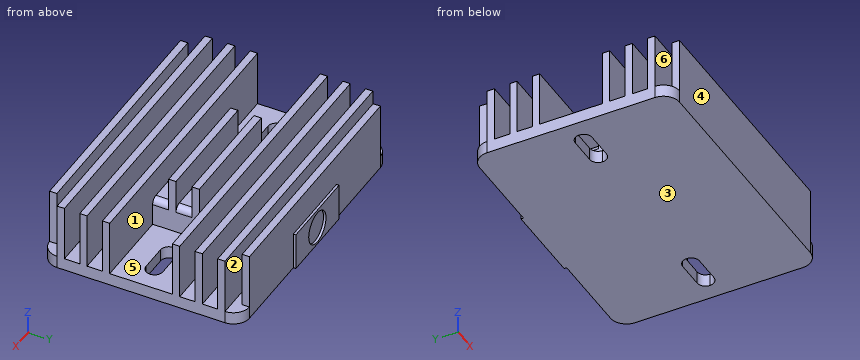
from build123d import *

# Parameters (mm, degrees)
SKETCH_1_W          = 110.2
SKETCH_1_H          = 79.6
EXTRUDE_1_DEPTH     = 4.99
SKETCH_2_W          = 52.2
SKETCH_2_H          = 6.4
EXTRUDE_2_DEPTH     = 15
SKETCH_3_W          = 46.2
SKETCH_3_H          = 73.2
EXTRUDE_3_DEPTH     = 11.2
SKETCH_4_W          = 97.6
SKETCH_4_H          = 2.9
SKETCH_4_W_2        = 46.2
SKETCH_4_W_3        = 110.2
EXTRUDE_4_DEPTH     = 22.4
SKETCH_5_W          = 17.339600334
SKETCH_5_H          = 6.7
CUT_EXTRUDE_1_DEPTH = 138.775034023
FILLET_1_R          = 3.3
FILLET_2_R          = 6.4
FILLET_3_R          = 2.5
SKETCH_6_W          = 32.2
SKETCH_6_H          = 15
EXTRUDE_5_DEPTH     = 1
SKETCH_7_R          = 6.438822501
CUT_EXTRUDE_2_DEPTH = 1


with BuildPart() as part:
    # ｽｹｯﾁ1 → ﾎﾞｽ - 押し出し1 (new body)
    with BuildSketch(Plane.XY):
        with Locations((55.1, 39.8)):
            Rectangle(SKETCH_1_W, SKETCH_1_H)
    extrude(amount=EXTRUDE_1_DEPTH)

    # ｽｹｯﾁ2 → ﾎﾞｽ - 押し出し2 (add)
    with BuildSketch(Plane.XY.offset(4.99)):
        with Locations((55.1, 76.4)):
            Rectangle(SKETCH_2_W, SKETCH_2_H)
    extrude(amount=EXTRUDE_2_DEPTH)

    # ｽｹｯﾁ3 → ﾎﾞｽ - 押し出し3 (add)
    with BuildSketch(Plane.XY.offset(4.99)):
        with Locations((55.1, 36.6)):
            Rectangle(SKETCH_3_W, SKETCH_3_H)
    extrude(amount=EXTRUDE_3_DEPTH)

    # ｽｹｯﾁ4 → ﾎﾞｽ - 押し出し4 (add)
    with BuildSketch(Plane.XY.offset(4.99)):
        with Locations((55.1, 78.15)):
            Rectangle(SKETCH_4_W, SKETCH_4_H)
        with Locations((55.1, 1.45)):
            Rectangle(SKETCH_4_W, SKETCH_4_H)
        with Locations((55.1, 44.45)):
            Rectangle(SKETCH_4_W_2, SKETCH_4_H)
        with Locations((55.1, 35.15)):
            Rectangle(SKETCH_4_W_2, SKETCH_4_H)
        with Locations((55.1, 53.75)):
            Rectangle(SKETCH_4_W_3, SKETCH_4_H)
        with Locations((55.1, 25.85)):
            Rectangle(SKETCH_4_W_3, SKETCH_4_H)
        with Locations((55.1, 71.781871857)):
            Rectangle(SKETCH_4_W_3, SKETCH_4_H)
        with Locations((55.1, 7.818128143)):
            Rectangle(SKETCH_4_W_3, SKETCH_4_H)
        with Locations((55.1, 16.834064072)):
            Rectangle(SKETCH_4_W_3, SKETCH_4_H)
        with Locations((55.1, 62.765935928)):
            Rectangle(SKETCH_4_W_3, SKETCH_4_H)
    extrude(amount=EXTRUDE_4_DEPTH)

    # ｽｹｯﾁ5 → ｶｯﾄ - 押し出し1 (cut, through all)
    with BuildSketch(Plane.XY.offset(4.99)):
        with Locations((15.05636048, 39.95)):
            Rectangle(SKETCH_5_W, SKETCH_5_H)
        with Locations((95.14363952, 39.95)):
            Rectangle(SKETCH_5_W, SKETCH_5_H)
    extrude(amount=-CUT_EXTRUDE_1_DEPTH, mode=Mode.SUBTRACT)

    # ﾌｨﾚｯﾄ1
    fillet_1_edges = [part.edges().sort_by_distance(p)[0] for p in [
        (6.386560313, 36.6, 2.495),
        (6.386560313, 43.3, 2.495),
        (23.726160647, 43.3, 2.495),
        (23.726160647, 36.6, 2.495),
        (86.473839353, 43.3, 2.495),
        (103.813439687, 43.3, 2.495),
        (103.813439687, 36.6, 2.495),
        (86.473839353, 36.6, 2.495),
    ]]
    fillet(fillet_1_edges, radius=FILLET_1_R)

    # ﾌｨﾚｯﾄ2
    fillet_2_edges = [part.edges().sort_by_distance(p)[0] for p in [
        (0, 0, 2.495),
        (110.2, 0, 2.495),
        (110.2, 79.6, 2.495),
        (0, 79.6, 2.495),
    ]]
    fillet(fillet_2_edges, radius=FILLET_2_R)

    # ﾌｨﾚｯﾄ3
    fillet_3_edges = [part.edges().sort_by_distance(p)[0] for p in [
        (78.2, 49.1, 16.19),
        (32, 39.8, 16.19),
        (78.2, 58.257967964, 16.19),
        (32, 49.1, 16.19),
        (78.2, 30.5, 16.19),
        (32, 21.342032036, 16.19),
        (81.2, 74.965935928, 19.99),
        (32, 67.273903893, 16.19),
        (78.2, 12.326096107, 16.19),
        (32, 4.634064072, 16.19),
        (32, 12.326096107, 16.19),
        (78.2, 21.342032036, 16.19),
        (78.2, 67.273903893, 16.19),
        (32, 58.257967964, 16.19),
        (29, 74.965935928, 19.99),
        (78.2, 4.634064072, 16.19),
        (32, 30.5, 16.19),
        (78.2, 39.8, 16.19),
    ]]
    fillet(fillet_3_edges, radius=FILLET_3_R)

    # ｽｹｯﾁ6 → ﾎﾞｽ - 押し出し5 (add)
    with BuildSketch(Plane(origin=(0, 79.6, 0), x_dir=(1, 0, 0), z_dir=(0, 1, 0))):
        with Locations((55.1, -7.5)):
            Rectangle(SKETCH_6_W, SKETCH_6_H)
    extrude(amount=EXTRUDE_5_DEPTH)

    # ｽｹｯﾁ7 → ｶｯﾄ - 押し出し2 (cut)
    with BuildSketch(Plane(origin=(0, 80.6, 0), x_dir=(1, 0, 0), z_dir=(0, 1, 0))):
        with Locations(Location((55.154186251, -7.301022377, 0), (0, 0, 270))):
            Circle(SKETCH_7_R)
    extrude(amount=-CUT_EXTRUDE_2_DEPTH, mode=Mode.SUBTRACT)


solid = part.part
CAD build for the part. Positions are in the model's coordinates, mm. Face numbers are marked on the shaded views. A direction names the side the tool comes from. Give positions to 0.01 mm unless a question says otherwise; leave off trailing zeros. Write each loop counter-clockwise with the first axis right and the second up, starting at its lowest first coordinate (ties: lowest second). Pieces come first, ordered by that corner, then holes. Notation, with made-up numbers: (-7, 79) -> (12, 79) arc R23 ccw to (12, 98) -> close; hole circle Ø5 at (51, 13). An arc over 180 degrees is marked (long way). Return JSON: item names as keys, results as strings.
Item 1: Two-plate mould, pull along Y, no slides. Class the marked faces 1, 2, 3 and 4: +Y half, -Y half, draft (parallel to the pull), parting line (faces both ways), or undercut.
Answer below:
{"face 1": "undercut", "face 2": "undercut", "face 3": "draft", "face 4": "-Y half"}
Item 2: Drill centre lines: probe 1 along Y at (x, z) = (6, 13.25); probe 2 along Y at (x, z) = (53.5, 2.5); probe 3 along X at (y, z) = (60, 12.5). Where is each one in solid material? Low to high.
Answer below:
{"probe 1": "y = 6.37 to 9.27, 15.38 to 18.28, 24.4 to 27.3, 52.3 to 55.2, 61.32 to 64.22, 70.33 to 73.23", "probe 2": "y = 0 to 79.6", "probe 3": "x = 32 to 78.2"}
Item 3: Drop flat-ended pins along their axis: pin 1 (1.7 mm diameter, centred on y = 4.5, z = 9.5, fed in from -X); pin 2 (1.5 mm diameter, centred on x = 87.5, z = 3.5, fed in from +Y); pin 3 (5 mm diameter, centred on x = 88.5, y = 21, fed in from +Z). Give the stop position or say it passes through.
Answer below:
{"pin 1": "stops at x = 32", "pin 2": "stops at y = 79.6", "pin 3": "stops at z = 4.99"}
Item 4: Band-saw the part on A-A (y = 31.5). List the corners of the cut face in (x, z), then the cut area to 3 significant figures.
Answer below:
{"outline": "(0, 0) -> (110.2, 0) -> (110.2, 4.99) -> (78.2, 4.99) -> (78.2, 13.69) arc R2.5 ccw to (75.7, 16.19) -> (34.5, 16.19) arc R2.5 ccw to (32, 13.69) -> (32, 4.99) -> (0, 4.99) -> close", "area": "1,060 mm2"}
Item 5: Tool access for the marked faces 5 and 6: list every direction of +Z, -Z, +X, -X, +Y, -Y with a clear straight run to the whole face (end or side of a thin tool).
Answer below:
{"face 5": "+Z, +X", "face 6": "+Z"}
Item 6: Band-saw the part on B-B (z = 23). Give the number of separate pieces and of enclosed holes in the cut face, then the cut area to 3 significant figures.
Answer below:
{"separate pieces": "10", "enclosed holes": "0", "area": "2,750 mm2"}
